```python
from build123d import *

# Parameters (mm, degrees)
SKETCH1_W           = 150
SKETCH1_H           = 120
BOSS_EXTRUDE1_DEPTH = 50
FILLET1_R           = 20
SHELL1_T            = -5
RIB1_REACH          = 110.282
SKETCH2_WALLS_W     = 358.564078278
SKETCH2_WALLS_H     = 5
SKETCH2_WALLS_W_2   = 360.016478266
SKETCH2_WALLS_W_3   = 5
SKETCH2_WALLS_H_2   = 328.564078278


with BuildPart() as part:
    # Sketch1 → Boss-Extrude1 (new body)
    with BuildSketch(Plane(origin=(0, 0, 0), x_dir=(1, 0, 0), z_dir=(0, 1, 0))):
        Rectangle(SKETCH1_W, SKETCH1_H)
    extrude(amount=BOSS_EXTRUDE1_DEPTH)

    # Fillet1
    fillet1_edges = [part.edges().sort_by_distance(p)[0] for p in [
        (-75, 50, 0),
        (0, 50, 60),
        (75, 50, 0),
        (0, 50, -60),
    ]]
    fillet(fillet1_edges, radius=FILLET1_R)

    # Shell1
    shell1_openings = [part.faces().sort_by_distance(p)[0] for p in [
        (0, 0, 0),
    ]]
    offset(amount=SHELL1_T, openings=shell1_openings)

    # Sketch2 walls → Rib1 (add, up to next)
    with BuildSketch(Plane.XZ, mode=Mode.PRIVATE) as rib1_sk1:
        with Locations((0, -28.619344042)):
            Rectangle(SKETCH2_WALLS_W, SKETCH2_WALLS_H)
    rib1_tool1 = extrude(rib1_sk1.sketch, amount=-RIB1_REACH, mode=Mode.PRIVATE) - part.part
    # Sketch2 walls → Rib1 (add, up to next)
    with BuildSketch(Plane.XZ, mode=Mode.PRIVATE) as rib1_sk2:
        Rectangle(SKETCH2_WALLS_W, SKETCH2_WALLS_H)
    rib1_tool2 = extrude(rib1_sk2.sketch, amount=-RIB1_REACH, mode=Mode.PRIVATE) - part.part
    # Sketch2 walls → Rib1 (add, up to next)
    with BuildSketch(Plane.XZ, mode=Mode.PRIVATE) as rib1_sk3:
        with Locations((0.726199994, 26.711483804)):
            Rectangle(SKETCH2_WALLS_W_2, SKETCH2_WALLS_H)
    rib1_tool3 = extrude(rib1_sk3.sketch, amount=-RIB1_REACH, mode=Mode.PRIVATE) - part.part
    # Sketch2 walls → Rib1 (add, up to next)
    with BuildSketch(Plane.XZ, mode=Mode.PRIVATE) as rib1_sk4:
        Rectangle(SKETCH2_WALLS_W_3, SKETCH2_WALLS_H_2)
    rib1_tool4 = extrude(rib1_sk4.sketch, amount=-RIB1_REACH, mode=Mode.PRIVATE) - part.part
    # Sketch2 walls → Rib1 (add, up to next)
    with BuildSketch(Plane.XZ, mode=Mode.PRIVATE) as rib1_sk5:
        Polygon((-34.534707577, 164.241613139), (-30.373449631, -164.304936346), (-25.37385063, -164.241613139), (-29.535108576, 164.304936346), align=None)
    rib1_tool5 = extrude(rib1_sk5.sketch, amount=-RIB1_REACH, mode=Mode.PRIVATE) - part.part
    # Sketch2 walls → Rib1 (add, up to next)
    with BuildSketch(Plane.XZ, mode=Mode.PRIVATE) as rib1_sk6:
        with Locations((39.408287459, 0)):
            Rectangle(SKETCH2_WALLS_W_3, SKETCH2_WALLS_H_2)
    rib1_tool6 = extrude(rib1_sk6.sketch, amount=-RIB1_REACH, mode=Mode.PRIVATE) - part.part
    add(rib1_tool1.solids().sort_by_distance((0, 0, -28.619344042))[0])
    add(rib1_tool2.solids().sort_by_distance((0, 0, 0))[0])
    add(rib1_tool3.solids().sort_by_distance((0.726199994, 0, 26.711483804))[0])
    add(rib1_tool4.solids().sort_by_distance((0, 0, 0))[0])
    add(rib1_tool5.solids().sort_by_distance((-29.954279104, 0, 0))[0])
    add(rib1_tool6.solids().sort_by_distance((39.408287459, 0, 0))[0])


solid = part.part
```
CAD build for the part. Positions are in the model's coordinates, mm. Round coordinates to 2 decimals unless told otherwise and drop trailing zeros. Order: outer loops, then holes, each group sorted by start corner. A loop starts at its lowest first (then second) coordinate and runs counter-clockwise, first axis right, second up.
Item 1: Saw through at B-B on z = -38. Write the cut outline in (x, y), then the cut area to 3 significant figures.
Item 2: Probe line 1 along Z through (x, y) = (-18, 8.5); line 2 along X through (y, z) = (10, 4); line 3 along X through (y, z) = (11.5, 54.5). List the from-to ranges inside material, lowest first.
Item 3: Saw through at C-C on y = 23. State how many separate pieces and enclosed holes the cut face has, then the cut area to 3 significant figures.
Item 4: Saw through at A-A on x = 19. Write the cut outline in (y, z), then the cut area to 3 significant figures.
Item 5: Saw through at D-D on z = 27. Write the cut outline in (x, y).
Item 6: Pin check, flat tips, straight feed: pin 1 (5 mm diameter, centred on x = 12.5, z = -4.5, fed in from -Y); pin 2 (5.5 mm diameter, centred on x = 46, z = 35, fed in from -Y); pin 3 (5 mm diameter, centred on y = 41.5, z = 37.5, fed in from +X); pin 4 (12 mm diameter, centred on x = -14.5, z = 40, fed in from -Y). Stop position of each tip, or through.
Item 7: Mould opens along Z. For faces 1 (the face through (75, 15, 1)), 2 (the face through (56, 15, -55)), 3 (the face through (-1, 15, 60)) say: pulls with the +Z half, pulls with the -Z half, needs draft (parallel to the pull), parting line crosses it, or undercut.
Reported:
1. outline: (-75, 0) - (-70, 0) - (-70, 30) arc R15 cw to (-55, 45) - (-31.97, 45) - (-31.97, 0) - (-26.97, 0) - (-26.97, 45) - (-2.5, 45) - (-2.5, 0) - (2.5, 0) - (2.5, 45) - (36.91, 45) - (36.91, 0) - (41.91, 0) - (41.91, 45) - (55, 45) arc R15 cw to (70, 30) - (70, 0) - (75, 0) - (75, 30) arc R20 ccw to (55, 50) - (-55, 50) arc R20 ccw to (-75, 30) - close
1. area: 1,800 mm2
2. line 1: z = -60 to -55, -31.12 to -26.12, -2.5 to 2.5, 24.21 to 29.21, 55 to 60
2. line 2: x = -75 to -70, -32.51 to -27.5, -2.5 to 2.5, 36.91 to 41.91, 70 to 75
2. line 3: x = -75 to -70, -33.14 to -28.14, -2.5 to 2.5, 36.91 to 41.91, 70 to 75
3. separate pieces: 1
3. enclosed holes: 16
3. area: 6,130 mm2
4. outline: (0, -60) - (30, -60) arc R20 ccw to (50, -40) - (50, 40) arc R20 ccw to (30, 60) - (0, 60) - (0, 55) - (30, 55) arc R15 cw to (45, 40) - (45, 29.21) - (0, 29.21) - (0, 24.21) - (45, 24.21) - (45, 2.5) - (0, 2.5) - (0, -2.5) - (45, -2.5) - (45, -26.12) - (0, -26.12) - (0, -31.12) - (45, -31.12) - (45, -40) arc R15 cw to (30, -55) - (0, -55) - close
4. area: 1,650 mm2
5. outline: (-75, 0) - (75, 0) - (75, 30) arc R20 ccw to (55, 50) - (-55, 50) arc R20 ccw to (-75, 30) - close
6. pin 1: stops at y = 0
6. pin 2: stops at y = 45
6. pin 3: stops at x = 72.86
6. pin 4: stops at y = 43.75
7. face 1: needs draft
7. face 2: undercut
7. face 3: pulls with the +Z half
